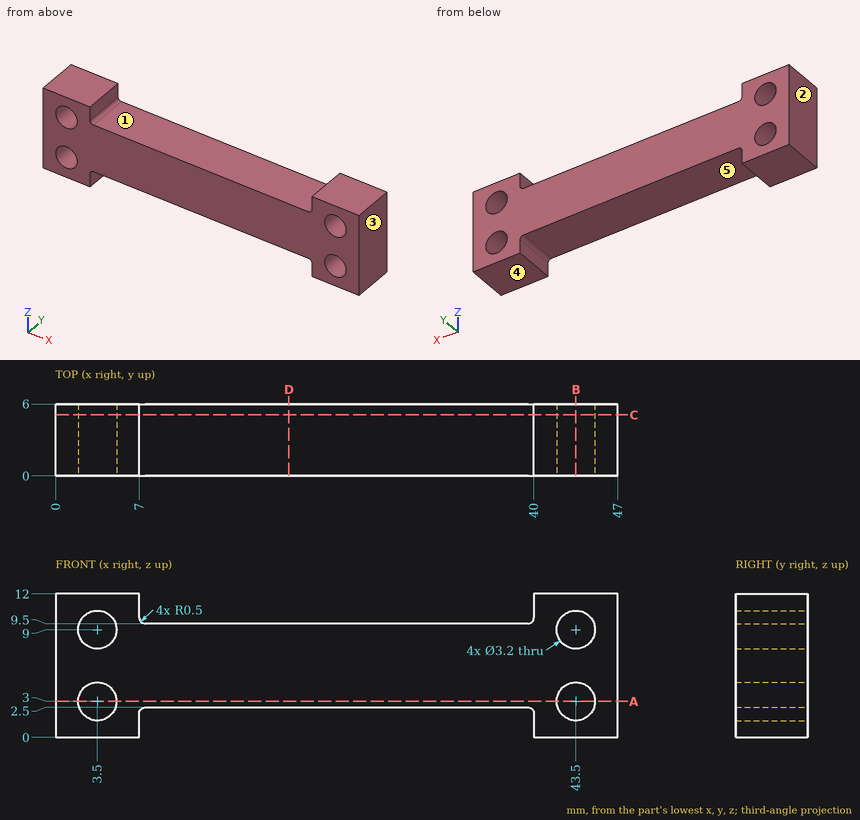
Can you work these out from the drawing? Everything is in mm from the part's minimum corner. A direction names the side the tool comes from. Coordinates: 2 decimals unless noted, no trailing zeros. Loops run counter-clockwise (first coordinate to the right, second up) from the corner with the lowest first, then second, coordinate; pieces in that order, holes last. Notation, with made-up numbers: (-27.5, -34) -> (-4.5, -34) arc R18 ccw to (-4.5, -5) -> close; hole circle Ø3 at (6.5, 25.25). An arc over 180 degrees is marked (long way). Return JSON: item names as keys, results as strings.
1) Thinking about a two-plate mould opening in X: for the marked faces 3, 4 and 5, which applies, +X half, -X half, draft (parallel to the pull), parting line (faces both ways), or undercut?
Results below:
{"face 3": "+X half", "face 4": "draft", "face 5": "undercut"}
2) If we section it at A-A, the plane z = 3: Write out the boundary of the cut face in (x, y).
Results below:
{"outline": "(0, 0) -> (1.9, 0) -> (1.9, 6) -> (0, 6) -> close; (5.1, 0) -> (41.9, 0) -> (41.9, 6) -> (5.1, 6) -> close; (45.1, 0) -> (47, 0) -> (47, 6) -> (45.1, 6) -> close"}
3) If we section it at B-B, the plane x = 43.5: Write out the boundary of the cut face in (y, z).
Results below:
{"outline": "(0, 0) -> (6, 0) -> (6, 1.4) -> (0, 1.4) -> close; (0, 4.6) -> (6, 4.6) -> (6, 7.4) -> (0, 7.4) -> close; (0, 10.6) -> (6, 10.6) -> (6, 12) -> (0, 12) -> close"}
4) Will these pins go through, and if not, where does the flat tip stop? pin 1 (3 mm diameter, centred on x = 25, y = 3.5, fed in from -Z); pin 2 (1.9 mm diameter, centred on x = 43.5, z = 3, fed in from +Y); pin 3 (3 mm diameter, centred on x = 37, y = 2.5, fed in from +Z).
Results below:
{"pin 1": "z = 2.5", "pin 2": "through", "pin 3": "z = 9.5"}
5) If we section it at C-C, the plane y = 5.1: Write out the boundary of the cut face in (x, z), then the cut area to 3 significant figures.
Results below:
{"outline": "(0, 0) -> (7, 0) -> (7, 2) arc R0.5 cw to (7.5, 2.5) -> (39.5, 2.5) arc R0.5 cw to (40, 2) -> (40, 0) -> (47, 0) -> (47, 12) -> (40, 12) -> (40, 10) arc R0.5 cw to (39.5, 9.5) -> (7.5, 9.5) arc R0.5 cw to (7, 10) -> (7, 12) -> (0, 12) -> close; hole circle Ø3.2 at (3.5, 3); hole circle Ø3.2 at (3.5, 9); hole circle Ø3.2 at (43.5, 3); hole circle Ø3.2 at (43.5, 9)", "area": "367 mm²"}
6) For the marked faces 1 and 2, which set-ups out of +Z, -Z, +X, -X, +Y, -Y let a thin tool reach every point of the face, with its end or its side?
Results below:
{"face 1": "+Z, +Y, -Y", "face 2": "+Z, -Z, -X, +Y, -Y"}
7) If we section it at D-D, the plane x = 19.5: Write out the boundary of the cut face in (y, z), then the cut area to 3 significant figures.
Results below:
{"outline": "(0, 2.5) -> (6, 2.5) -> (6, 9.5) -> (0, 9.5) -> close", "area": "42.0 mm²"}
8) I need wall thicknesses on line 1 (X direction, y = 4.7, z = 9); line 2 (Z direction, x = 43.5, y = 2.95); line 3 (X direction, y = 3.95, z = 0.75). Which ranges of each line are inside material? Lowest first, please. Write a range as from..to.
Results below:
{"line 1": "0..1.9, 5.1..41.9, 45.1..47", "line 2": "0..1.4, 4.6..7.4, 10.6..12", "line 3": "0..7, 40..47"}
